from build123d import *

# Parameters (mm, degrees)
BOSS_EXTRUDE1_DEPTH = 3
SKETCH2_R           = 5
BOSS_EXTRUDE2_DEPTH = 1.5
FILLET1_R           = 2


with BuildPart() as part:
    # Sketch1 → Boss-Extrude1 (new body)
    with BuildSketch(Plane(origin=(0, 0, 0), x_dir=(1, 0, 0), z_dir=(0, 1, 0))):
        with BuildLine():
            Line((-5, 0), (-5, 37))
            ThreePointArc((-5, 37), (0, 42), (5, 37))
            Line((5, 37), (5, 0))
            ThreePointArc((5, 0), (0, -5), (-5, 0))
        make_face()
    extrude(amount=BOSS_EXTRUDE1_DEPTH)

    # Sketch2 → Boss-Extrude2 (add)
    with BuildSketch(Plane(origin=(0, 3, 0), x_dir=(1, 0, 0), z_dir=(0, 1, 0))):
        with BuildLine():
            ThreePointArc((-5, 0), (0, -5), (5, 0))
            ThreePointArc((5, 0), (0, 5), (-5, 0))
        make_face()
        with Locations(Location((0, 37, 0), (0, 0, 180))):
            Circle(SKETCH2_R)
    extrude(amount=BOSS_EXTRUDE2_DEPTH)

    # Fillet1
    fillet1_edges = [part.edges().sort_by_distance(p)[0] for p in [
        (-5, 0, -18.5),
        (0, 0, -42),
        (5, 0, -18.5),
        (0, 0, 5),
    ]]
    fillet(fillet1_edges, radius=FILLET1_R)


solid = part.part
Input: part model. Units: mm. Frame: model coordinates. A direction names the side the tool comes from. Round coordinates to 2 decimals unless told otherwise and drop trailing zeros. Order: outer loops, then holes, each group sorted by start corner. A loop starts at its lowest first (then second) coordinate and runs counter-clockwise, first axis right, second up. Notation, with made-up numbers: (19, 18.25) - (78, 18.25) arc R21 ccw to (78, 42.25) - close; hole circle Ø10 at (3.5, 30). An arc over 180 degrees is marked (long way). Answer as a JSON object with one key per item and string values. Group by question number.
(1) Material intervals for probe 1 along Y at (x, z) = (-3, -17); probe 2 along Z at (x, y) = (-3, 3.8); probe 3 along Z at (x, y) = (3.5, 3.9), sorted ascending. Write a range as from..to.
(2) Pin query (flat end, axial travel): P1, Ø1, axis at x = -4, y = 3.5, coming from the +Z side; P2, Ø1, axis at y = 4, z = -12, coming from the +X side. Return the tip coordinate at first contact, or that it passes through.
(3) Cut plane B-B (y = 3.6). Return loops of the section in (x, z), then the cut area to 3 significant figures.
(4) Cut plane A-A (x = 0). Return loops of the section in (y, z).
(5) Draft query along Z for faces 1 (the face through (0, 3, -19)), 2 (the face through (-4.43, 0.6, -18.76)), 3 (the face through (1.08, 3.51, -41.88)). Return one class per face: released by +Z, released by -Z, zero draft, split by the parting line, or undercut.
(6) Cut plane C-C (z = -9.5). Return loops of the section in (x, y).
(7) Reachability of faces 4 (the face through (0, 4.5, 0)), 5 (the face through (-1.08, 3.51, 4.88)) from +Z, -Z, +X, -X, +Y, -Y: full face, straight path, thin tool, end or side. Return the list, or none.
Here are the results:
{
 "1": {"probe 1": "y = 0..3", "probe 2": "z = -41..-33, -4..4", "probe 3": "z = -40.57..-33.43, -3.57..3.57"},
 "2": {"P1": "stops at z = 3.57", "P2": "passes through"},
 "3": {"outline": "circle Ø10 at (0, -37); circle Ø10 at (0, 0)", "area": "157 mm^2"},
 "4": {"outline": "(0, -40) arc R2 ccw to (2, -42) - (4.5, -42) - (4.5, -32) - (3, -32) - (3, -5) - (4.5, -5) - (4.5, 5) - (2, 5) arc R2 ccw to (0, 3) - close"},
 "5": {"face 1": "undercut", "face 2": "zero draft", "face 3": "undercut"},
 "6": {"outline": "(-5, 2) arc R2 ccw to (-3, 0) - (3, 0) arc R2 ccw to (5, 2) - (5, 3) - (-5, 3) - close"},
 "7": {"face 4": "+Z, -Z, +X, -X, +Y", "face 5": "+Y"}
}
